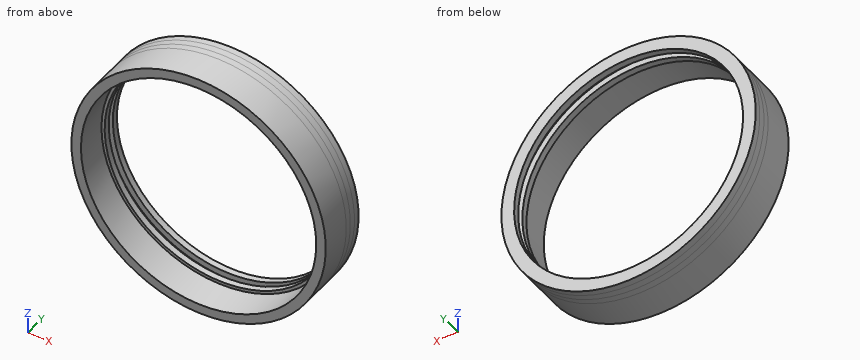
from build123d import *

# Parameters (mm, degrees)
SKETCH1_R           = 20
SKETCH1_R_2         = 18
BOSS_EXTRUDE1_DEPTH = 1
BOSS_EXTRUDE2_START = 1
SKETCH2_R           = 20
SKETCH2_R_2         = 19
BOSS_EXTRUDE2_DEPTH = 1
BOSS_EXTRUDE3_START = 1
SKETCH3_R           = 20
SKETCH3_R_2         = 18
BOSS_EXTRUDE3_DEPTH = 1
BOSS_EXTRUDE4_START = 5
SKETCH4_R           = 20
SKETCH4_R_2         = 18.5
BOSS_EXTRUDE4_DEPTH = 5


with BuildPart() as part:
    # Sketch1 → Boss-Extrude1 (new body)
    with BuildSketch(Plane(origin=(0, 0, 0), x_dir=(1, 0, 0), z_dir=(0, 1, 0))):
        with Locations(Location((0, 0, 0), (0, 0, 270))):
            Circle(SKETCH1_R)
        with Locations(Location((0, 0, 0), (0, 0, 270))):
            Circle(SKETCH1_R_2, mode=Mode.SUBTRACT)
    extrude(amount=BOSS_EXTRUDE1_DEPTH)

    # Sketch2 → Boss-Extrude2 (add)
    with BuildSketch(Plane.XZ.offset(BOSS_EXTRUDE2_START)):
        with Locations(Location((0, 0, 0), (0, 0, 270))):
            Circle(SKETCH2_R)
        with Locations(Location((0, 0, 0), (0, 0, 270))):
            Circle(SKETCH2_R_2, mode=Mode.SUBTRACT)
    extrude(amount=-BOSS_EXTRUDE2_DEPTH)

    # Sketch3 → Boss-Extrude3 (add)
    with BuildSketch(Plane.XZ.offset(1).offset(BOSS_EXTRUDE3_START)):
        with Locations(Location((0, 0, 0), (0, 0, 270))):
            Circle(SKETCH3_R)
        with Locations(Location((0, 0, 0), (0, 0, 90))):
            Circle(SKETCH3_R_2, mode=Mode.SUBTRACT)
    extrude(amount=-BOSS_EXTRUDE3_DEPTH)

    # Sketch4 → Boss-Extrude4 (add)
    with BuildSketch(Plane.XZ.offset(2).offset(BOSS_EXTRUDE4_START)):
        with Locations(Location((0, 0, 0), (0, 0, 270))):
            Circle(SKETCH4_R)
        with Locations(Location((0, 0, 0), (0, 0, 270))):
            Circle(SKETCH4_R_2, mode=Mode.SUBTRACT)
    extrude(amount=-BOSS_EXTRUDE4_DEPTH)


solid = part.part
Could you check a few things on this model? Use its own coordinates, in mm. Round coordinates to 2 decimals unless told otherwise and drop trailing zeros. Order: outer loops, then holes, each group sorted by start corner. A loop starts at its lowest first (then second) coordinate and runs counter-clockwise, first axis right, second up.
(1) Imagine slicing it at C-C (y = -1.5). Write out the boundary of the cut face in (x, z), plus the area to 3 significant figures.
Response values:
outline: circle Ø40 at (0, 0); hole circle Ø36 at (0, 0)
area: 239 mm2
(2) Imagine slicing it at A-A (z = 0). Write out the boundary of the cut face in (x, y), plus the area to 3 significant figures.
Response values:
outline: (-20, -7) - (-18.5, -7) - (-18.5, -2) - (-18, -2) - (-18, -1) - (-19, -1) - (-19, 0) - (-18, 0) - (-18, 1) - (-20, 1) - close; (18, -2) - (18.5, -2) - (18.5, -7) - (20, -7) - (20, 1) - (18, 1) - (18, 0) - (19, 0) - (19, -1) - (18, -1) - close
area: 25.0 mm2
(3) I'm going to push flat-ended pins straight in: pin 1 (1.5 mm diameter, centred on y = -3.5, z = -5.5, fed in from -X); pin 2 (2 mm diameter, centred on y = -5.5, z = 12, fed in from -X). Where does each tip first touch, or does it pass through?
Response values:
pin 1: stops at x = -19.43
pin 2: stops at x = -16.7
(4) Please list where these lines run through material, in increasing order: line 1 along X through (y, z) = (-0.35, 0); line 2 along Y through (x, z) = (13, -13); line 3 along X through (y, z) = (0.55, 0).
Response values:
line 1: x = -20 to -19, 19 to 20
line 2: y = -2 to -1, 0 to 1
line 3: x = -20 to -18, 18 to 20
(5) Imagine slicing it at B-B (x = 0). Write out the boundary of the cut face in (y, z).
Response values:
outline: (-7, -20) - (1, -20) - (1, -18) - (0, -18) - (0, -19) - (-1, -19) - (-1, -18) - (-2, -18) - (-2, -18.5) - (-7, -18.5) - close; (-7, 18.5) - (-2, 18.5) - (-2, 18) - (-1, 18) - (-1, 19) - (0, 19) - (0, 18) - (1, 18) - (1, 20) - (-7, 20) - close
